Input: part model. Units: mm. Frame: model coordinates. A direction names the side the tool comes from. Give positions to 0.01 mm unless a question says otherwise; leave off trailing zeros. Loops run counter-clockwise (first coordinate to the right, second up) from the corner with the lowest first, then second, coordinate; pieces in that order, holes last. Notation, with made-up numbers: M 53.5,12 L 68.5,12 A36 cw 68.5,46 Z; hole C 42.25,31 d8. An arc over 180 degrees is marked long. Answer as a JSON object with one key per item and string values. Group by question number.
1) Section query D-D on z = 9.5. Return loops of the section in (x, y).
2) Section query B-B on z = -63.5. Return loops of the section in (x, y), plus the area to 3 significant figures.
3) Section query A-A on y = 131. Return loops of the section in (x, z).
4) Section query C-C on x = -11. Return loops of the section in (y, z), plus the area to 3 significant figures.
5) First-contact query: P1, Ø20, axis at x = -3.5, y = -29, coming from the -Z side; P2, Ø21, axis at x = -133.5, z = -79, coming from the +Y side; P3, Ø2, axis at x = 88, z = -47.5, coming from the +Y side. Flat tips, straight axial feed; report the tip coordinate or a pass-through.
6) Access query for faces 5 (the flat face through (-129, 42, -90)), 6 (the flat face through (96, 101, 4)), 7 (the flat face through (-129, 50, -90)), 8 (the flat face through (118, 50, -68)), 9 (the flat face through (-1, 6, 24)). Directions: +Z, -Z, +X, -X, +Y, -Y. A direction counts if a zero-diameter tool reaches every point of the face in a straight line with its end or side. Return the directions, or none.
7) Draft query along X for faces 1 (the flat face through (-118, 50, -69)), 2 (the flat face through (-122, 50, -68)), 3 (the cylindrical face through (-106.594, 49.79, -12.028)), 4 (the flat face through (-99, 223.942, -88)). Return one class per face: +X half, -X half, draft (parallel to the pull), parting line (faces both ways), or undercut.
8) Ray query, L1, parallel to X at y = 232.5, z = -99; L2, parallel to Z at x = -13, y = -8.5; L3, parallel to Y at x = -96, z = -89. Return the intervals inside material, ascending.
from build123d import *

# Parameters (mm, degrees)
EXTRUDE_1_DEPTH     = 4
SKETCH_11_W         = 156
SKETCH_11_H         = 90
EXTRUDE_2_DEPTH     = 20
SKETCH_12_W         = 38
SKETCH_12_H         = 4
SKETCH_14_W         = 38
SKETCH_14_H         = 50
EXTRUDE_3_DEPTH     = 20
SKETCH_16_W         = 238.183586275
SKETCH_16_H         = 132.295328182
CUT_EXTRUDE_1_DEPTH = 10
SKETCH_17_W         = 40
SKETCH_17_H         = 20
EXTRUDE_4_DEPTH     = 4
SKETCH_21_R         = 6
EXTRUDE_8_DEPTH     = 4
EXTRUDE_11_DEPTH    = 15
EXTRUDE_12_DEPTH    = 8


with BuildPart() as part:
    # 草图1 → 凸台-拉伸1 (new body)
    with BuildSketch(Plane.XY):
        Polygon((-40, 0), (40, 0), (40, -160), (78, -160), (78, 0), (78, 50), (118, 90), (80, 90), (40, 50), (-40, 50), (-80, 90), (-118, 90), (-78, 50), (-78, 0), (-78, -160), (-40, -160), align=None)
    extrude(amount=EXTRUDE_1_DEPTH)

    # 草图11 → 凸台-拉伸2 (add)
    with BuildSketch(Plane.XY.offset(4)):
        with Locations((0, 5)):
            Rectangle(SKETCH_11_W, SKETCH_11_H)
    extrude(amount=EXTRUDE_2_DEPTH)

    # 扫描1: sweep along a path in 草图13
    with BuildLine(Plane(origin=(78, 0, 0), x_dir=(0, 0, -1), z_dir=(1, 0, 0))) as sweep_1_path:
        Line((-4, 90), (-4, 150))
        Line((-4, 150), (41, 227.942286341))
        Line((41, 227.942286341), (131, 227.942286341))
    # 草图12 → 扫描1 (sweep)
    with BuildSketch(Plane(origin=(0, 90, 0), x_dir=(1, 0, 0), z_dir=(0, 1, 0))):
        with Locations((-99, -2)):
            Rectangle(SKETCH_12_W, SKETCH_12_H)
        with Locations((99, -2)):
            Rectangle(SKETCH_12_W, SKETCH_12_H)
    sweep(path=sweep_1_path.line, transition=Transition.RIGHT)

    # 草图14 → 凸台-拉伸3 (add)
    with BuildSketch(Plane(origin=(0, 227.942286341, 0), x_dir=(1, 0, 0), z_dir=(0, 1, 0))):
        with Locations((-99, 106)):
            Rectangle(SKETCH_14_W, SKETCH_14_H)
        with Locations((99, 106)):
            Rectangle(SKETCH_14_W, SKETCH_14_H)
    extrude(amount=EXTRUDE_3_DEPTH)

    # 草图16 → 切除-拉伸1 (cut)
    with BuildSketch(Plane(origin=(0, 0, 0), x_dir=(-1, 0, 0), z_dir=(0, 0, -1))):
        with Locations((8.714033644, -106.147664091)):
            Rectangle(SKETCH_16_W, SKETCH_16_H)
    extrude(amount=-CUT_EXTRUDE_1_DEPTH, mode=Mode.SUBTRACT)

    # 草图17 → 凸台-拉伸4 (add)
    with BuildSketch(Plane.XZ.offset(40)):
        with Locations((0, 10)):
            Rectangle(SKETCH_17_W, SKETCH_17_H)
    extrude(amount=EXTRUDE_4_DEPTH)

    # 草图21 → 凸台-拉伸8 (add)
    with BuildSketch(Plane.XZ.offset(44)):
        with Locations((0, 9.5)):
            Circle(SKETCH_21_R)
    extrude(amount=EXTRUDE_8_DEPTH)

    # 草图28 → 凸台-拉伸11 (add, symmetric)
    with BuildSketch(Plane(origin=(0, 50, 0), x_dir=(1, 0, 0), z_dir=(0, 1, 0))):
        with BuildLine():
            Line((-122, 40), (-122, 97))
            Line((-122, 97), (-118, 97))
            Line((-118, 97), (-118, 40))
            ThreePointArc((-118, 40), (-106.284271247, 11.715728753), (-78, 0))
            Line((-78, 0), (-78, -4))
            ThreePointArc((-78, -4), (-109.112698372, 8.887301628), (-122, 40))
        make_face()
        with BuildLine():
            Line((118, 40), (118, 97))
            Line((118, 97), (122, 97))
            Line((122, 97), (122, 40))
            ThreePointArc((122, 40), (109.112698372, 8.887301628), (78, -4))
            Line((78, -4), (78, 0))
            ThreePointArc((78, 0), (106.284271247, 11.715728753), (118, 40))
        make_face()
    extrude(amount=EXTRUDE_11_DEPTH, both=True)

    # 草图29 → 凸台-拉伸12 (add)
    with BuildSketch(Plane(origin=(0, 50, 0), x_dir=(1, 0, 0), z_dir=(0, 1, 0))):
        Polygon((122, 97), (148, 97), (122, 71), align=None)
        Polygon((-122, 97), (-148, 97), (-122, 71), align=None)
    extrude(amount=-EXTRUDE_12_DEPTH)


solid = part.part
Output:
{
 "1": {"outline": "M -78,-40 L -20,-40 L -20,-44 L -6,-44 L -6,-48 L 6,-48 L 6,-44 L 20,-44 L 20,-40 L 78,-40 L 78,50 L -78,50 Z"},
 "2": {"outline": "M -122,35 L -118,35 L -118,65 L -122,65 Z; M -118,223.94 L -80,223.94 L -80,227.94 L -118,227.94 Z; M 80,223.94 L 118,223.94 L 118,227.94 L 80,227.94 Z; M 118,35 L 122,35 L 122,65 L 118,65 Z", "area": "544 mm^2"},
 "3": {"outline": "M -118,0 L -80,0 L -80,4 L -118,4 Z; M 80,0 L 118,0 L 118,4 L 80,4 Z"},
 "4": {"outline": "M -44,0 L -40,0 L -40,4 L 0,4 L 0,0 L 50,0 L 50,24 L -40,24 L -40,20 L -44,20 Z", "area": "2,080 mm^2"},
 "5": {"P1": "stops at z = 4", "P2": "stops at y = 50", "P3": "stops at y = 227.94"},
 "6": {"face 5": "+Z, -Z, -X, -Y", "face 6": "+Z, +X, -X, +Y", "face 7": "+Z, -Z, -X, +Y", "face 8": "-Z, -Y", "face 9": "+Z, +X, -X, +Y, -Y"},
 "7": {"face 1": "undercut", "face 2": "-X half", "face 3": "undercut", "face 4": "draft"},
 "8": {"L1": "x = -118 to -80, 80 to 118", "L2": "z = 4 to 24", "L3": "y = 223.94 to 247.94"}
}
